Could you check a few things on this model? Use its own coordinates, in mm. Coordinates: 2 decimals unless noted, no trailing zeros. Loops run counter-clockwise (first coordinate to the right, second up) from the corner with the lowest first, then second, coordinate; pieces in that order, holes last.
Autodesk Fusion 360 part; units mm, degrees
sketch "Sketch1" plane through (0, 0, 0) normal (0, 0, 1) x (1, 0, 0) in component "Pneumatic Nut"
  line L0 (-3, 5.1962) -> (-6, 0)
  line L1 (-6, 0) -> (-3, -5.1962)
  line L2 (-3, -5.1962) -> (3, -5.1962)
  line L3 (3, -5.1962) -> (6, 0)
  line L4 (6, 0) -> (3, 5.1962)
  line L5 (3, 5.1962) -> (-3, 5.1962)
  circle A0 centre (0, 0) radius 2.775
  dimension "d1" = 12
  dimension "d2" = 5.55
extrude "Extrude1" add sketch "Sketch1" along normal blind 5 in component "Pneumatic Nut"
chamfer "Chamfer1" distance 1 angle 45 6 edges at (4.5, -2.5981, 5) (4.5, 2.5981, 5) (0, 5.1962, 5) (-4.5, 2.5981, 5) (-4.5, -2.5981, 5) (0, -5.1962, 5) in component "Pneumatic Nut"
component "Pneumatic Nut" placed x (1, 0, 0) y (0, 1, 0) z (0, 0, 1) at (0, 0, 0)
1) Imagine slicing it at D-D on x = 4. List the corners of the cut face in (y, z) for me, plus the area to 3 significant figures.
2) If I drill on L1, parallel to Y at x = 0, z = 2.5 (3 decimals); L2, parallel to Y at x = -1, z = 2.5; L3, parallel to X at y = 2.5, z = 4.8, over which ranges is the centre line in solid material (lowest first)?
3) Imagine slicing it at C-C on y = 2.25. List the corners of the cut face in (x, z) for me.
4) Imagine slicing it at A-A on z = 3.1. List the corners of the cut face in (x, y) for me (3 decimals), plus the area to 3 significant figures.
5) Will these pins go through, and if not, where does the flat tip stop? pin 1 (1.5 mm diameter, centred on x = 3.5, z = 1, fed in from +Y); pin 2 (1.5 mm diameter, centred on y = -1.5, z = 4, fed in from -X); pin 3 (2 mm diameter, centred on x = -4.5, z = 3, fed in from -Y); pin 4 (1.5 mm diameter, centred on y = 1, z = 1, fed in from +X).
6) We'd pull the mould along Y, two halves only. Please class faces 1 (the flat face through (0, 3, 5)), 2 (the cylindrical face through (1.49, -2.34, 2.46)), 3 (the flat face through (0, -5.196, 2)), 4 (the flat face through (-4.08, 2.31, 4.51)): released by +Y, released by -Y, zero draft, split by the parting line, or undercut.
7) Imagine slicing it at B-B on x = 0. List the corners of the cut face in (y, z) for me (3 decimals), plus the area to 3 significant figures.
Solved:
1. outline: (-3.46, 0) - (3.46, 0) - (3.46, 4) - (1.46, 5) - (-1.46, 5) - (-3.46, 4) - close
1. area: 32.6 mm2
2. L1: y = -5.196 to -2.775, 2.775 to 5.196
2. L2: y = -5.2 to -2.59, 2.59 to 5.2
2. L3: x = -3.63 to -1.2, 1.2 to 3.63
3. outline: (-4.7, 0) - (-1.62, 0) - (-1.62, 5) - (-3.55, 5) - (-4.7, 4) - close; (1.62, 0) - (4.7, 0) - (4.7, 4) - (3.55, 5) - (1.62, 5) - close
4. outline: (-6, 0) - (-3, -5.196) - (3, -5.196) - (6, 0) - (3, 5.196) - (-3, 5.196) - close; hole circle Ø5.55 at (0, 0)
4. area: 69.3 mm2
5. pin 1: stops at y = 5.2
5. pin 2: stops at x = -5.57
5. pin 3: stops at y = -4.33
5. pin 4: stops at x = 5.86
6. face 1: zero draft
6. face 2: undercut
6. face 3: released by -Y
6. face 4: released by +Y
7. outline: (-5.196, 0) - (-2.775, 0) - (-2.775, 5) - (-4.196, 5) - (-5.196, 4) - close; (2.775, 0) - (5.196, 0) - (5.196, 4) - (4.196, 5) - (2.775, 5) - close
7. area: 23.2 mm2
